Part print with two shaded views. Sizes in mm from the minimum x, y, z corner. A direction names the side the tool comes from. Coordinates: 2 decimals unless noted, no trailing zeros. Loops run counter-clockwise (first coordinate to the right, second up) from the corner with the lowest first, then second, coordinate; pieces in that order, holes last. Notation, with made-up numbers: (62, 51.5) - (92, 51.5) arc R32 ccw to (92, 85.5) - close; hole circle Ø1 at (-30, -32). An arc over 180 degrees is marked (long way). Answer as CSV lines item,"result".
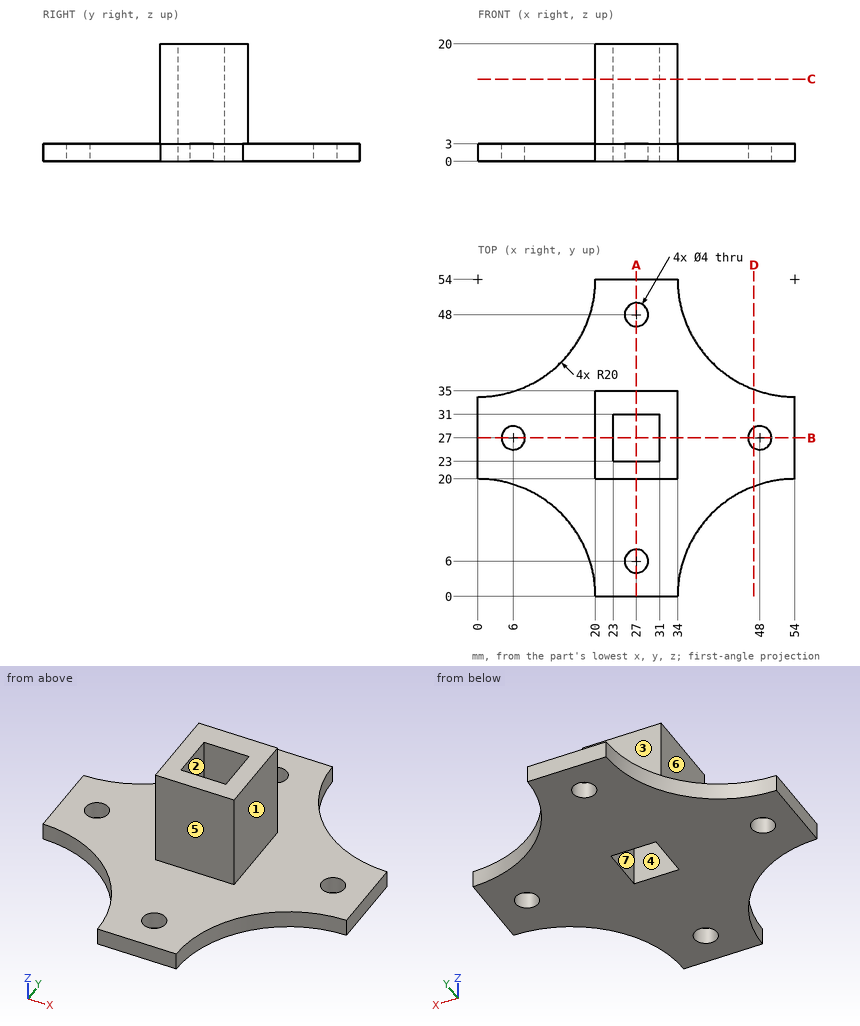
Q1. Two-plate mould, pull along Y, no slides. Class the marked faces 1, 2, 3 and 4: released by +Y, released by -Y, zero draft, split by the parting line, or undercut.
Results:
face 1,"zero draft"
face 2,"undercut"
face 3,"released by +Y"
face 4,"undercut"
Q2. Saw through at D-D (x = 47). Give the cut face in (y, z) (3 decimals).
Results:
outline,"(18.735, 0) - (25.268, 0) - (25.268, 3) - (18.735, 3) - close; (28.732, 0) - (35.265, 0) - (35.265, 3) - (28.732, 3) - close"
Q3. Saw through at A-A (x = 27). Give the cut face in (y, z), then the cut area to 3 significant figures.
Results:
outline,"(0, 0) - (4, 0) - (4, 3) - (0, 3) - close; (8, 0) - (23, 0) - (23, 20) - (20, 20) - (20, 3) - (8, 3) - close; (31, 0) - (46, 0) - (46, 3) - (35, 3) - (35, 20) - (31, 20) - close; (50, 0) - (54, 0) - (54, 3) - (50, 3) - close"
area,"233 mm^2"
Q4. Which spindle directions (+Z, -Z, +X, -X, +Y, -Y) get a long thin tool onto all of the face, cutting with end or side? Do the marked faces 5, 6 and 7. Say none if no direction does.
Results:
face 5,"+Z, +X, -X, -Y"
face 6,"+Z, -X, +Y, -Y"
face 7,"+Z, -Z"
Q5. Saw through at C-C (z = 14). Give the cut face in (x, y).
Results:
outline,"(20, 20) - (34, 20) - (34, 35) - (20, 35) - close; hole (23, 23) - (31, 23) - (31, 31) - (23, 31) - close"
Q6. Flat gauge pins, fed straight in: pin 1 (8 mm diameter, centred on x = 17, y = 26, fed in from +Z); pin 2 (2 mm diameter, centred on y = 10.5, z = 2.5, fed in from -X); pin 3 (12 mm diameter, centred on y = 26.5, z = 15.5, fed in from -X); pin 4 (12 mm diameter, centred on x = 46, y = 31, fed in from +Z). Where does each tip first touch, or does it go through?
Results:
pin 1,"stops at z = 20"
pin 2,"stops at x = 16.36"
pin 3,"stops at x = 20"
pin 4,"stops at z = 3"
Q7. Saw through at B-B (y = 27). Give the cut face in (x, z), then the cut area to 3 significant figures.
Results:
outline,"(0, 0) - (4, 0) - (4, 3) - (0, 3) - close; (8, 0) - (23, 0) - (23, 20) - (20, 20) - (20, 3) - (8, 3) - close; (31, 0) - (46, 0) - (46, 3) - (34, 3) - (34, 20) - (31, 20) - close; (50, 0) - (54, 0) - (54, 3) - (50, 3) - close"
area,"216 mm^2"
Q8. Wall check: L1, parallel to Y at x = 27, z = 1.6; L2, parallel to X at y = 30, z = 17; L3, parallel to Y at x = 26, z = 1.5. Give the ranges that are in metal, low to high.
Results:
L1,"y = 0 to 4, 8 to 23, 31 to 46, 50 to 54"
L2,"x = 20 to 23, 31 to 34"
L3,"y = 0 to 4.27, 7.73 to 23, 31 to 46.27, 49.73 to 54"
